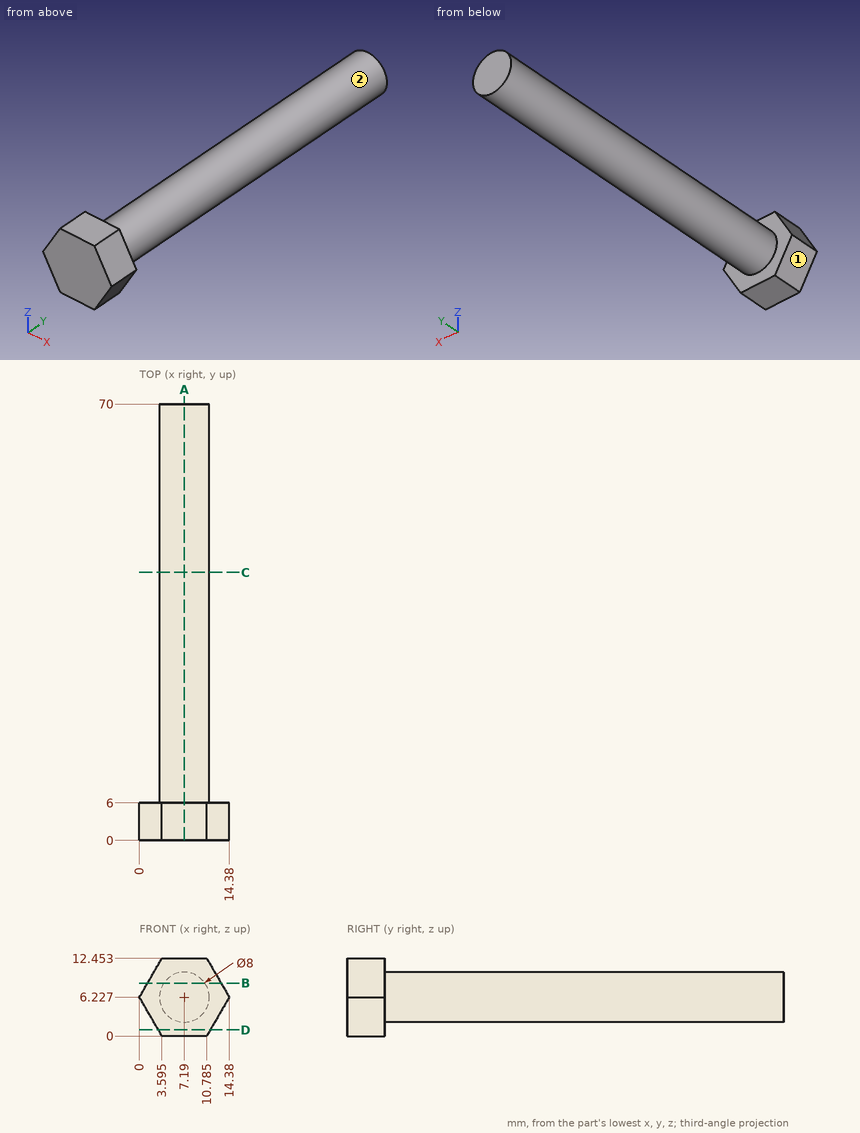
Print and shaded views of the part. All mm, measured from the part's lowest x, y and z. A direction names the side the tool comes from. Coordinates: 2 decimals unless noted, no trailing zeros. Order: outer loops, then holes, each group sorted by start corner. A loop starts at its lowest first (then second) coordinate and runs counter-clockwise, first axis right, second up. Notation, with made-up numbers: M 24.25,28.25 L 72.25,28.25 A17 ccw 72.25,50.25 Z; hole C 79,78 d6. An arc over 180 degrees is marked long. Write each question's results on one line, items separated by ' | '. Start each with the question number.
Q1. Which spindle directions (+Z, -Z, +X, -X, +Y, -Y) get a long thin tool onto all of the face, cutting with end or side? Do the marked faces 1 and 2. Say none if no direction does.
Q2. Cut at A-A (x = 7.19). List the corners of the cut face in (y, z).
Q3. Drill centre lines: probe 1 along Y at (x, z) = (3, 5.5); probe 2 along X at (y, z) = (59.5, 8) (1 decimal); probe 3 along Z at (x, y) = (3.5, 58) (1 decimal). Where is each one in solid material? Low to high. Write a range as from..to.
Q4. Cut at C-C (y = 43). List the corners of the cut face in (x, z).
Q5. Flat gauge pins, fed straight in: P1, Ø5, axis at x = 12.5, y = 23.5, coming from the -Z side; P2, Ø3, axis at y = 59.5, z = 5.5, coming from the -X side; P3, Ø3, axis at x = 2, y = 14, coming from the +Z side. Where does each tip first touch, or does it go through?
Q6. Cut at B-B (z = 8.5). List the corners of the cut face in (x, y).
Q7. Cut at D-D (z = 1). List the corners of the cut face in (x, y).
Found:
1) face 1: -Z, -X, +Y, -Y | face 2: +Y
2) outline: M 0,0 L 6,0 L 6,2.23 L 70,2.23 L 70,10.23 L 6,10.23 L 6,12.45 L 0,12.45 Z
3) probe 1: 0..6 | probe 2: 3.6..10.8 | probe 3: 4.7..7.8
4) outline: C 7.19,6.23 d8
5) P1: z = 3.38 | P2: x = 3.19 | P3: z = 7.77
6) outline: M 1.31,0 L 13.07,0 L 13.07,6 L 10.48,6 L 10.48,70 L 3.9,70 L 3.9,6 L 1.31,6 Z
7) outline: M 3.02,0 L 11.36,0 L 11.36,6 L 3.02,6 Z
